Work out the finished part from the listing and answer in its coordinate system (mm). A direction names the side the tool comes from. Round coordinates to 2 decimals unless told otherwise and drop trailing zeros. Loops run counter-clockwise (first coordinate to the right, second up) from the corner with the lowest first, then second, coordinate; pieces in that order, holes last.
```python
from build123d import *

# Parameters (mm, degrees)
SKETCH1_W           = 95
SKETCH1_H           = 72
SKETCH1_R           = 1.25
BOSS_EXTRUDE1_DEPTH = 14.2
FILLET1_R           = 0.5
FILLET2_R           = 1
SKETCH2_W           = 93
SKETCH2_H           = 70
CUT_EXTRUDE1_DEPTH  = 1.6
SKETCH3_W           = 93
SKETCH3_H           = 70
CUT_EXTRUDE2_DEPTH  = 1.6


with BuildPart() as part:
    # Sketch1 → Boss-Extrude1 (new body)
    with BuildSketch(Plane(origin=(0, 0, 0), x_dir=(1, 0, 0), z_dir=(0, 1, 0))):
        Rectangle(SKETCH1_W, SKETCH1_H)
        with Locations(Location((-44, 32.5, 0), (0, 0, 270))):
            Circle(SKETCH1_R, mode=Mode.SUBTRACT)
        with Locations(Location((44, 32.5, 0), (0, 0, 90))):
            Circle(SKETCH1_R, mode=Mode.SUBTRACT)
        with Locations(Location((44, -32.5, 0), (0, 0, 270))):
            Circle(SKETCH1_R, mode=Mode.SUBTRACT)
        with Locations(Location((-44, -32.5, 0), (0, 0, 90))):
            Circle(SKETCH1_R, mode=Mode.SUBTRACT)
        with BuildLine():
            Line((-44, 30), (-46.5, 30))
            Line((-46.5, 30), (-46.5, -30))
            Line((-46.5, -30), (-44, -30))
            ThreePointArc((-44, -30), (-42.232233047, -30.732233047), (-41.5, -32.5))
            Line((-41.5, -32.5), (-41.5, -35))
            Line((-41.5, -35), (41.5, -35))
            Line((41.5, -35), (41.5, -32.5))
            ThreePointArc((41.5, -32.5), (42.232233047, -30.732233047), (44, -30))
            Line((44, -30), (46.5, -30))
            Line((46.5, -30), (46.5, 30))
            Line((46.5, 30), (44, 30))
            ThreePointArc((44, 30), (42.232233047, 30.732233047), (41.5, 32.5))
            Line((41.5, 32.5), (41.5, 35))
            Line((41.5, 35), (-41.5, 35))
            Line((-41.5, 35), (-41.5, 32.5))
            ThreePointArc((-41.5, 32.5), (-42.232233047, 30.732233047), (-44, 30))
        make_face(mode=Mode.SUBTRACT)
    extrude(amount=BOSS_EXTRUDE1_DEPTH)

    # Fillet1
    fillet1_edges = [part.edges().sort_by_distance(p)[0] for p in [
        (47.5, 7.1, -36),
        (47.5, 7.1, 36),
        (-47.5, 7.1, 36),
        (-47.5, 7.1, -36),
    ]]
    fillet(fillet1_edges, radius=FILLET1_R)

    # Fillet2
    fillet2_edges = [part.edges().sort_by_distance(p)[0] for p in [
        (-46.5, 7.1, -30),
        (-46.5, 7.1, 30),
        (-41.5, 7.1, 35),
        (41.5, 7.1, 35),
        (46.5, 7.1, 30),
        (46.5, 7.1, -30),
        (41.5, 7.1, -35),
        (-41.5, 7.1, -35),
    ]]
    fillet(fillet2_edges, radius=FILLET2_R)

    # Sketch2 → Cut-Extrude1 (cut)
    with BuildSketch(Plane(origin=(0, 14.2, 0), x_dir=(1, 0, 0), z_dir=(0, 1, 0))):
        Rectangle(SKETCH2_W, SKETCH2_H)
    extrude(amount=-CUT_EXTRUDE1_DEPTH, mode=Mode.SUBTRACT)

    # Sketch3 → Cut-Extrude2 (cut)
    with BuildSketch(Plane.XZ):
        Rectangle(SKETCH3_W, SKETCH3_H)
    extrude(amount=-CUT_EXTRUDE2_DEPTH, mode=Mode.SUBTRACT)


solid = part.part
```
1. Which of the six approach directions +Z, -Z, +X, -X, +Y, -Y give full straight-line access (tool end or side, diameter ignored) to faces 4 (the face through (-44, 1.6, -34)), 5 (the face through (44, 12.6, 34)), 6 (the face through (42, 7, -31)), 7 (the face through (47.5, 7, 0))?
Answer key:
face 4: -Y
face 5: +Y
face 6: +Y, -Y
face 7: +Z, -Z, +X, +Y, -Y
2. Find section C-C (y = 11.5). Give the number of separate pieces and of enclosed holes in the cut face, then the cut area to 3 significant figures.
Answer key:
separate pieces: 1
enclosed holes: 5
area: 407 mm2
3. Determine the mould class of faces 1 (the face through (45.5, 1.6, 32.7)), 2 (the face through (-47.5, 7, 0)), 3 (the face through (-1, 7, 36)) for opening direction Z: +Z half, -Z half, draft (parallel to the pull), parting line (faces both ways), or undercut.
Answer key:
face 1: undercut
face 2: draft
face 3: +Z half
4. Find section B-B (x = 28). Write down the section's boundary in (y, z).
Answer key:
outline: (0, -36) - (14.2, -36) - (14.2, -35) - (0, -35) - close; (0, 35) - (14.2, 35) - (14.2, 36) - (0, 36) - close
5. Given pin 1 (3 mm diameter, centred on x = -43.5, z = 32.5, fed in from +Y); pin 2 (4 mm diameter, centred on x = 44, z = -32.5, fed in from -Y), each flat-ended and moving along its own axis, determine where each tip first touches the part or whether it passes through.
Answer key:
pin 1: stops at y = 12.6
pin 2: stops at y = 1.6
6. Find section A-A (z = -3.5). Write down the section's boundary in (x, y), then the cut area to 3 significant figures.
Answer key:
outline: (-47.5, 0) - (-46.5, 0) - (-46.5, 14.2) - (-47.5, 14.2) - close; (46.5, 0) - (47.5, 0) - (47.5, 14.2) - (46.5, 14.2) - close
area: 28.4 mm2
7. Consider probe 1 along X at (y, z) = (6.75, -32.5); probe 2 along X at (y, z) = (6.5, 9.5); probe 3 along Z at (x, y) = (-4, 10.75). Determine where each line is inside the solid, lowest interval first.
Answer key:
probe 1: x = -47.5 to -45.25, -42.75 to -41.5, 41.5 to 42.75, 45.25 to 47.5
probe 2: x = -47.5 to -46.5, 46.5 to 47.5
probe 3: z = -36 to -35, 35 to 36
